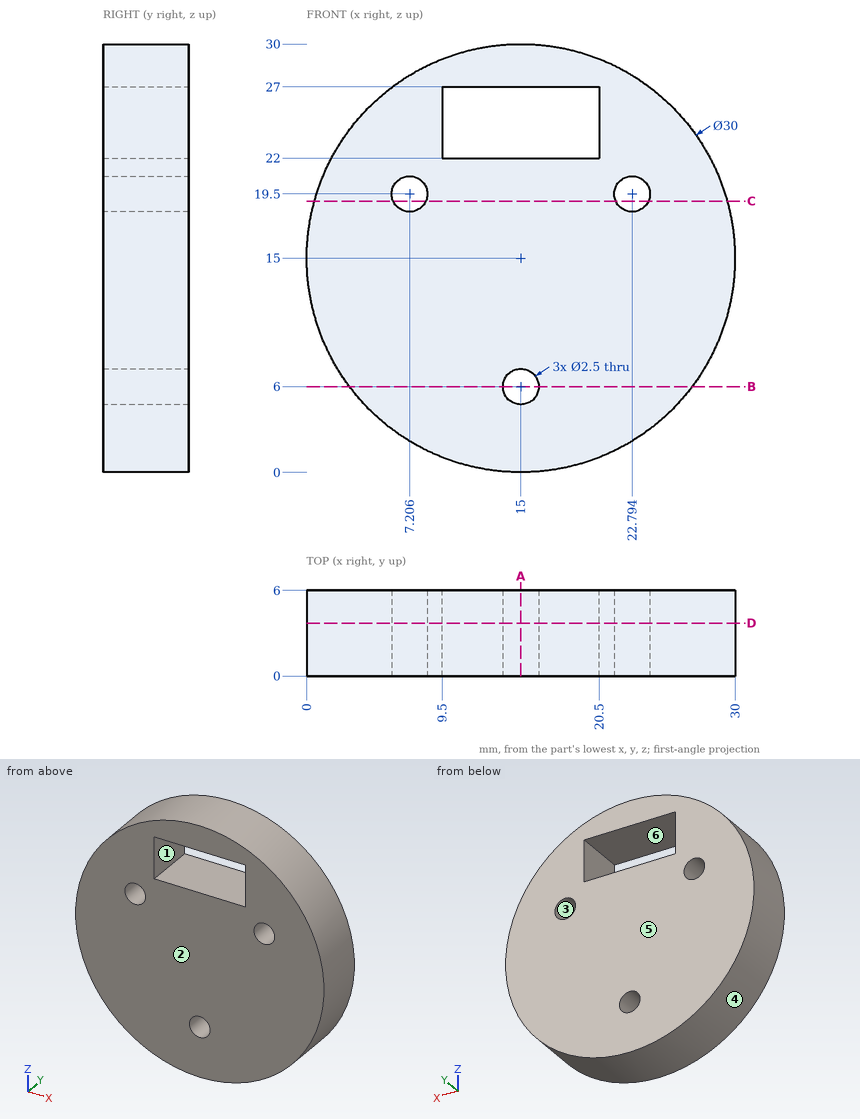
Here's the drawing with two shaded views (mm, measured from the low corner). I have some questions. A direction names the side the tool comes from. Coordinates: 2 decimals unless noted, no trailing zeros. Loops run counter-clockwise (first coordinate to the right, second up) from the corner with the lowest first, then second, coordinate; pieces in that order, holes last. Notation, with made-up numbers: M 6,-33 L 42,-33 A21 ccw 42,6 Z; hole C -22,75 d5. An arc over 180 degrees is marked long. Put each result on its own line as item: value. Start each with the question number.
(1) Imagine slicing it at D-D on y = 3.7. List the corners of the cut face in (x, z) for me, and give its area (3 significant figures).
(2) Which directions (+Z, -Z, +X, -X, +Y, -Y) give clear straight access to the entire face, cutting with the end or side of a thin tool? Please do the marked faces 5 and 6.
(3) Will these pins go through, and if not, where does the flat tip stop? pin 1 Ø2 at (x, z) = (22.79, 19.5) entering from -Y; pin 2 Ø2 at (x, y) = (19.5, 4.5) entering from +Z; pin 3 Ø1.5 at (x, y) = (18, 1.5) entering from +Z; pin 4 Ø1 at (y, z) = (3.5, 24) entering from +X.
(4) We'd pull the mould along Z, two halves only. Please class the marked faces 1, 2, 3 and 4: +Z half, -Z half, draft (parallel to the pull), parting line (faces both ways), or undercut.
(5) I need wall thicknesses on probe 1 along X at (y, z) = (4.15, 19.5); probe 2 along Z at (x, y) = (14.5, 2.6) (1 decimal); probe 3 along Z at (x, y) = (20.25, 3.25). Which ranges of each line are inside material? Lowest first, please.
(6) Imagine slicing it at C-C on z = 19. List the corners of the cut face in (x, y) for me, and give its area (3 significant figures).
(7) Imagine slicing it at A-A on x = 15. List the corners of the cut face in (y, z) for me, and give its area (3 significant figures).
(8) Imagine slicing it at B-B on z = 6. List the corners of the cut face in (x, y) for me.
Worked answers:
1. outline: C 15,15 d30; hole C 7.21,19.5 d2.5; hole M 9.5,22 L 20.5,22 L 20.5,27 L 9.5,27 Z; hole C 15,6 d2.5; hole C 22.79,19.5 d2.5
1. area: 637 mm2
2. face 5: +Z, -Z, +X, -X, +Y
2. face 6: +Y, -Y
3. pin 1: passes through
3. pin 2: stops at z = 29.59
3. pin 3: stops at z = 29.83
3. pin 4: stops at x = 27.36
4. face 1: undercut
4. face 2: draft
4. face 3: undercut
4. face 4: parting line
5. probe 1: x = 0.69 to 5.96, 8.46 to 21.54, 24.04 to 29.31
5. probe 2: z = 0 to 4.9, 7.1 to 22, 27 to 30
5. probe 3: z = 0.95 to 22, 27 to 29.05
6. outline: M 0.54,0 L 6.06,0 L 6.06,6 L 0.54,6 Z; M 8.35,0 L 21.65,0 L 21.65,6 L 8.35,6 Z; M 23.94,0 L 29.46,0 L 29.46,6 L 23.94,6 Z
6. area: 146 mm2
7. outline: M 0,0 L 6,0 L 6,4.75 L 0,4.75 Z; M 0,7.25 L 6,7.25 L 6,22 L 0,22 Z; M 0,27 L 6,27 L 6,30 L 0,30 Z
7. area: 135 mm2
8. outline: M 3,0 L 13.75,0 L 13.75,6 L 3,6 Z; M 16.25,0 L 27,0 L 27,6 L 16.25,6 Z
